Can you work these out from the model? Positions are in its coordinate system, mm. Face numbers are marked on the shaded views. Give positions to 0.01 mm unless a question says otherwise; leave off trailing zeros. Loops run counter-clockwise (first coordinate to the right, second up) from the corner with the lowest first, then second, coordinate; pieces in that order, holes last.
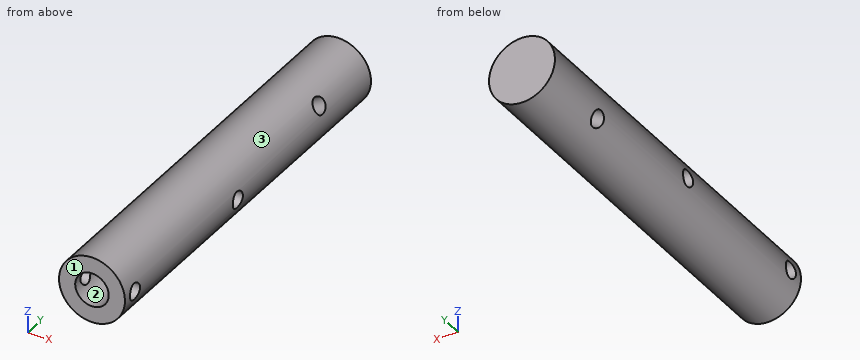
from build123d import *

# Parameters (mm, degrees)
TWELVE_MILLIMETRE_AXLE_STOCK_SKETCH_R = 6
TWELVE_MILLIMETRE_AXLE_STOCK_DEPTH    = 73
MOTOR_COUPLING_SOCKET_SKETCH_R        = 3.05
MOTOR_COUPLING_SOCKET_DEPTH           = 22.1
FRONT_COLLAR_PIN_SKETCH_R             = 1.5
FRONT_COLLAR_PIN_DEPTH                = 14
REAR_COLLAR_PIN_SKETCH_R              = 1.5
REAR_COLLAR_PIN_DEPTH                 = 14
HUB_DRIVE_PIN_SKETCH_R                = 1.5
HUB_DRIVE_PIN_DEPTH                   = 14


with BuildPart() as part:
    # Twelve millimetre axle stock sketch → Twelve millimetre axle stock (new body)
    with BuildSketch(Plane(origin=(0, -283, 0), x_dir=(1, 0, 0), z_dir=(0, 1, 0))):
        with Locations(Location((-19.009182883, 53.244882879, 0), (0, 0, 270))):
            Circle(TWELVE_MILLIMETRE_AXLE_STOCK_SKETCH_R)
    extrude(amount=TWELVE_MILLIMETRE_AXLE_STOCK_DEPTH)

    # Motor coupling socket sketch → Motor coupling socket (cut)
    with BuildSketch(Plane(origin=(0, -232, 0), x_dir=(1, 0, 0), z_dir=(0, 1, 0))):
        with Locations(Location((-19.009182883, 53.244882879, 0), (0, 0, 270))):
            Circle(MOTOR_COUPLING_SOCKET_SKETCH_R)
    extrude(amount=MOTOR_COUPLING_SOCKET_DEPTH, mode=Mode.SUBTRACT)

    # Front collar pin sketch → Front collar pin (cut)
    with BuildSketch(Plane(origin=(-26.009182883, 0, 0), x_dir=(0, 0, -1), z_dir=(1, 0, 0))):
        with Locations(Location((53.244882879, -213, 0), (0, 0, 180))):
            Circle(FRONT_COLLAR_PIN_SKETCH_R)
    extrude(amount=FRONT_COLLAR_PIN_DEPTH, mode=Mode.SUBTRACT)

    # Rear collar pin sketch → Rear collar pin (cut)
    with BuildSketch(Plane(origin=(-26.009182883, 0, 0), x_dir=(0, 0, -1), z_dir=(1, 0, 0))):
        with Locations(Location((53.244882879, -243.5, 0), (0, 0, 180))):
            Circle(REAR_COLLAR_PIN_SKETCH_R)
    extrude(amount=REAR_COLLAR_PIN_DEPTH, mode=Mode.SUBTRACT)

    # Hub drive pin sketch → Hub drive pin (cut)
    with BuildSketch(Plane(origin=(-43.374775586, 0, -25.042438361), x_dir=(0.5000000000000001, 0, -0.8660254037844386), z_dir=(0.8660254037844386, 0, 0.5000000000000001))):
        with Locations(Location((36.606829753, -269, 0), (0, 0, 180))):
            Circle(HUB_DRIVE_PIN_SKETCH_R)
    extrude(amount=HUB_DRIVE_PIN_DEPTH, mode=Mode.SUBTRACT)


with BuildPart() as body_2:
    # Mirror1: mirrored copy
    add(part.part.mirror(Plane(origin=(0, 0, 0), x_dir=(0, 0, 1), z_dir=(0, -1, 0))))


solid = body_2.part
(1) Will these pins go through, and if not, where does the flat tip stop? P1, Ø2.5, axis at y = 213, z = -53.24, coming from the -X side; P2, Ø5, axis at x = -23, y = 247, coming from the +Z side; P3, Ø1.5, axis at x = -21, y = 256.5, coming from the -Z side; P4, Ø3, axis at x = -19, z = -52, coming from the -Y side.
Returned:
P1: passes through
P2: stops at z = -47.43
P3: stops at z = -59.12
P4: stops at y = 232
(2) Suppose I cut it at A-A on y = 213. List the corners of the cut face in (x, z) for me, plus the area to 3 significant figures.
Returned:
outline: (-24.82, -54.74) arc R6 ccw to (-13.2, -54.74) - (-16.35, -54.74) arc R3.05 cw to (-21.66, -54.74) - close; (-24.82, -51.74) - (-21.66, -51.74) arc R3.05 cw to (-16.35, -51.74) - (-13.2, -51.74) arc R6 ccw to start
area: 65.8 mm2
(3) Please list where these lines run through material, in increasing order: probe 1 along Y at (x, z) = (-24.5, -54); probe 2 along Y at (x, z) = (-14.5, -53.75); probe 3 along X at (y, z) = (227, -55.5).
Returned:
probe 1: y = 210 to 211.7, 214.3 to 242.2, 244.8 to 283
probe 2: y = 210 to 211.59, 214.41 to 242.09, 244.91 to 283
probe 3: x = -24.57 to -21.06, -16.96 to -13.45
(4) Thinking about a two-plate mould opening in X: for the marked faces 1, 2 and 3, which applies, pulls with the +X half, pulls with the -X half, needs draft (parallel to the pull), parting line crosses it, or undercut?
Returned:
face 1: needs draft
face 2: undercut
face 3: parting line crosses it
(5) Suppose I cut it at D-D on y = 243.5. List the corners of the cut face in (x, z) for me, plus the area to 3 significant figures.
Returned:
outline: (-24.82, -54.74) arc R6 ccw to (-13.2, -54.74) - close; (-24.82, -51.74) - (-13.2, -51.74) arc R6 ccw to start
area: 77.5 mm2
(6) Suppose I cut it at B-B on z = -54. Give the number of separate pieces and of enclosed holes in the cut face, plus the area to 3 significant figures.
Returned:
separate pieces: 4
enclosed holes: 1
area: 678 mm2
